Geometry check sheet. Reference: drawing and pictorial views, mm from the part's lowest x, y, z. Coordinates: 2 decimals unless noted, no trailing zeros. Write each loop counter-clockwise with the first axis right and the second up, starting at its lowest first coordinate (ties: lowest second). Pieces come first, ordered by that corner, then holes. Notation, with made-up numbers: (86.5, -16) - (94.5, -16) arc R14 cw to (94.5, 4) - close; hole circle Ø3 at (66.25, 27). An arc over 180 degrees is marked (long way). Use one line per item in the form item = value. Start each with the question number.
(1) Mould release check, pull along Z, two halves, no side actions. Record for the marked faces 1, 2 and 3: released by +Z, released by -Z, zero draft, split by the parting line, or undercut.
(2) Sectioned sample at B-B (y = 0.5). Count the separate pieces of the cut face and the enclosed holes in it.
(3) Material ranges on line 1 (Y direction, x = 6.35, z = 1.15); line 2 (Z direction, x = 8.25, y = 4.25) (1 decimal); line 3 (X direction, y = 2, z = 10.5) (1 decimal), recorded low to high. Write a range as [from, to].
(4) Gauge pin test, flat ends, axial feed: pin 1 Ø2 at (x, y) = (2.5, 3) entering from -Z (1 decimal); pin 2 Ø1.5 at (x, y) = (9, 3) entering from -Z. Record the tip position at first contact, or that the pin passes through.
(5) Sectioned sample at A-A (x = 2.5). Record the cut outline in (y, z).
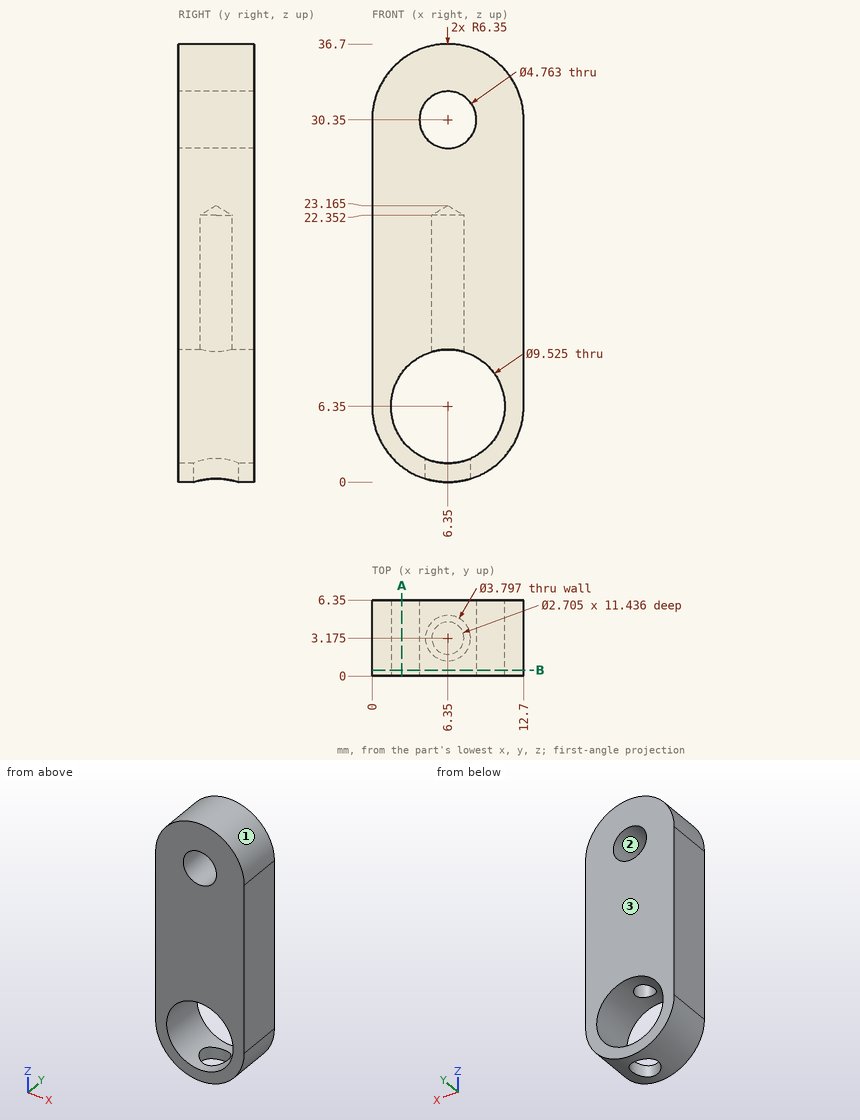
Answers below:
q1.face_1 = released by +Z
q1.face_2 = undercut
q1.face_3 = zero draft
q2.separate_pieces = 1
q2.enclosed_holes = 2
q3.line_1 = [0, 1.28], [5.07, 6.35]
q3.line_2 = [0.3, 2], [10.7, 28.9], [31.8, 36.4]
q3.line_3 = [0, 4], [8.7, 12.7]
q4.pin_1 = 0.7
q4.pin_2 = 0.29
q5.outline = (0, 1.3) - (6.35, 1.3) - (6.35, 3.55) - (0, 3.55) - close; (0, 9.15) - (6.35, 9.15) - (6.35, 35.4) - (0, 35.4) - close
